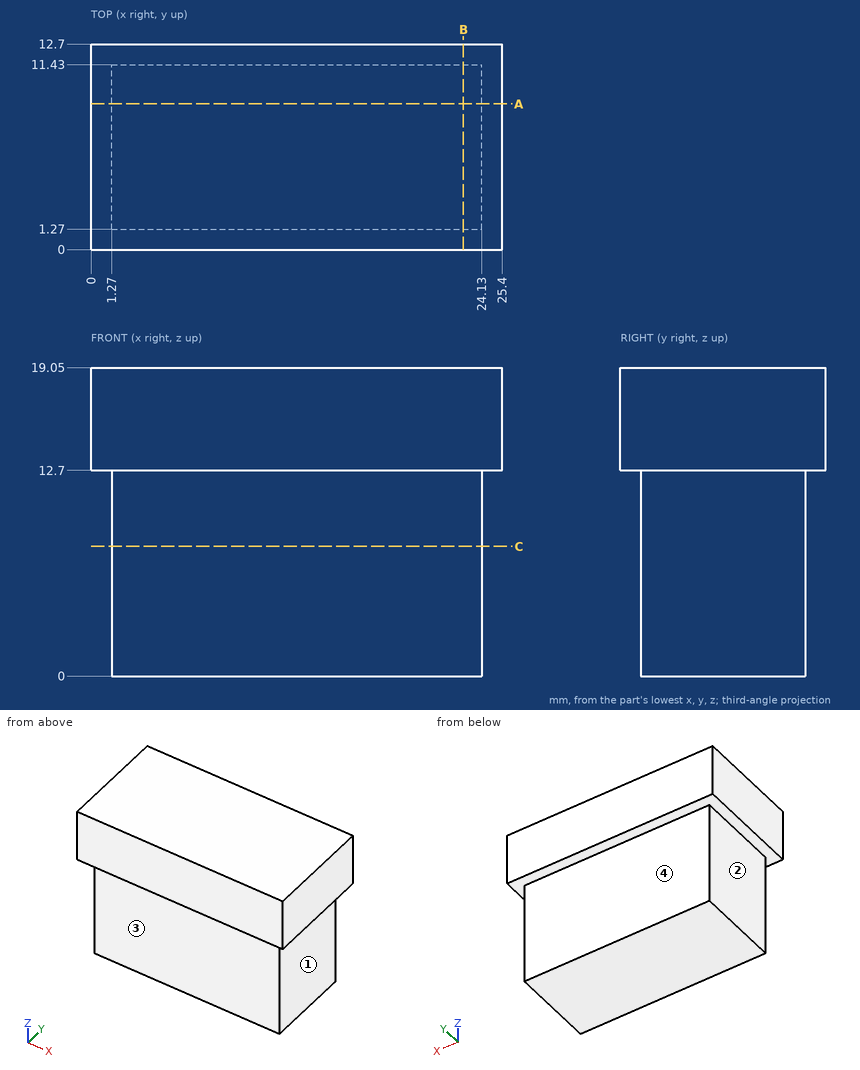
Input: dimensioned drawing with shaded views. Units: mm. Origin: part minimum x, y, z. A direction names the side the tool comes from. Coordinates: 2 decimals unless noted, no trailing zeros. Order: outer loops, then holes, each group sorted by start corner. A loop starts at its lowest first (then second) coordinate and runs counter-clockwise, first axis right, second up. Notation, with made-up numbers: (11.5, 70) - (42.5, 70) arc R28 ccw to (42.5, 91) - close; hole circle Ø9 at (48, 47.5). An arc over 180 degrees is marked (long way). Return JSON: item names as keys, results as strings. Group by question number.
1. Cut plane A-A (y = 9). Output: boundary loops of the cut face in (x, z).
2. Cut plane C-C (z = 8). Output: boundary loops of the cut face in (x, y).
3. Material intervals for line 1 along Y through (x, z) = (8.5, 9); line 2 along Z through (x, y) = (1, 2.75); line 3 along X through (y, z) = (5.25, 4.25), sorted ascending. Write a range as [from, to].
4. Cut plane B-B (x = 23). Output: boundary loops of the cut face in (y, z).
5. Pin query (flat end, axial travel): pin 1 (3 mm diameter, centred on y = 7.5, z = 8, fed in from +X); pin 2 (4 mm diameter, centred on x = 15.5, z = 7.5, fed in from +Y); pin 3 (3 mm diameter, centred on y = 6.5, z = 3.5, fed in from -X). Return the tip coordinate at first contact, or that it passes through.
6. Set-up query: the marked faces 1, 2, 3 and 4. Return all of +Z, -Z, +X, -X, +Y, -Y with unobstructed straight access to the full face (end or side cutting, diameter ignored); none if empty.
Resolved:
{
 "1": {"outline": "(0, 12.7) - (1.27, 12.7) - (1.27, 0) - (24.13, 0) - (24.13, 12.7) - (25.4, 12.7) - (25.4, 19.05) - (0, 19.05) - close"},
 "2": {"outline": "(1.27, 1.27) - (24.13, 1.27) - (24.13, 11.43) - (1.27, 11.43) - close"},
 "3": {"line 1": "y = [1.27, 11.43]", "line 2": "z = [12.7, 19.05]", "line 3": "x = [1.27, 24.13]"},
 "4": {"outline": "(0, 12.7) - (1.27, 12.7) - (1.27, 0) - (11.43, 0) - (11.43, 12.7) - (12.7, 12.7) - (12.7, 19.05) - (0, 19.05) - close"},
 "5": {"pin 1": "stops at x = 24.13", "pin 2": "stops at y = 11.43", "pin 3": "stops at x = 1.27"},
 "6": {"face 1": "-Z, +X, +Y, -Y", "face 2": "-Z, -X, +Y, -Y", "face 3": "-Z, +X, -X, -Y", "face 4": "-Z, +X, -X, +Y"}
}
